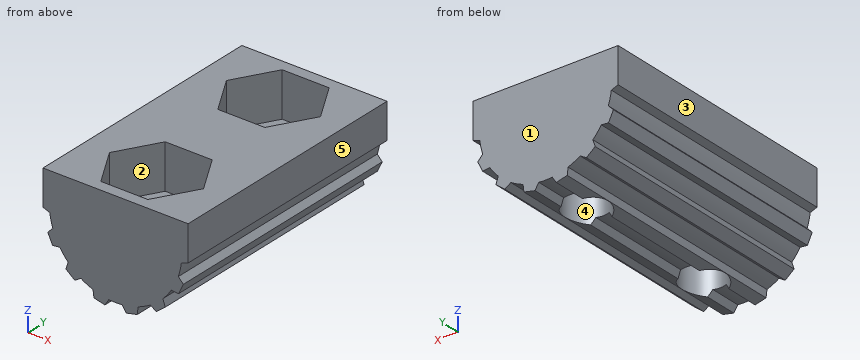
```python
from build123d import *

# Parameters (mm, degrees)
BOSS_EXTRUDE1_DEPTH             = 8.5
BOSS_EXTRUDE2_REACH             = 12.596
BOSS_EXTRUDE2_DIRECTION_2_REACH = 12.596
CIRPATTERN1_START               = -8.5
CIRPATTERN1_DEPTH               = 17
CUT_EXTRUDE1_DEPTH              = 19.347920123
CUT_EXTRUDE1_DEPTH_BACK         = 19.347920123
SKETCH10_W                      = 9.8
SKETCH10_H                      = 17
BOSS_EXTRUDE3_DEPTH             = 2
M2_5_CLEARANCE_HOLE1_D          = 2.9
CUT_EXTRUDE2_DEPTH              = 3


# Read off the part's stored shape, not the designer's step: CirPattern1
with BuildPart() as part:
    # Sketch1 → Boss-Extrude1 (new, symmetric)
    with BuildSketch(Plane(origin=(0, 0, 0), x_dir=(1, 0, 0), z_dir=(0, 1, 0))):
        with BuildLine():
            ThreePointArc((-4.44, 0.547426308), (-4.465207061, 0.274228857), (-4.473619962, 0))
            Line((-4.473619962, 0), (-4.44, 0))
            Line((-4.44, 0), (-4.44, 0.547426308))
        make_face()
        with BuildLine():
            Line((-4.44, 0.547426308), (-4.44, 0))
            Line((-4.44, 0), (4.473619962, 0))
            ThreePointArc((4.473619962, 0), (0.274228857, 4.465207061), (-4.44, 0.547426308))
        make_face()
    extrude(amount=BOSS_EXTRUDE1_DEPTH, both=True)

    # Boss-Extrude2: up to this face of the body (flat: up to its plane)
    boss_extrude2_end = Plane(part.part.faces().sort_by_distance((0, 8.5, -1.898663281))[0])
    # Sketch1<3> → Boss-Extrude2 (add, up to the picked face)
    with BuildSketch(Plane(origin=(0, 0, 0), x_dir=(1, 0, 0), z_dir=(0, 1, 0)), mode=Mode.PRIVATE) as boss_extrude2_sk1:
        Polygon((-4.44, 0.547426308), (-4.44, -0.547426308), (-4.9, -0.38), (-4.9, 0.38), align=None)
    boss_extrude2_tool1 = split(extrude(boss_extrude2_sk1.sketch, amount=BOSS_EXTRUDE2_REACH, mode=Mode.PRIVATE), bisect_by=boss_extrude2_end, keep=Keep.BOTH, mode=Mode.PRIVATE)
    # Sketch1<3> → Boss-Extrude2 (add, up to the picked face)
    with BuildSketch(Plane(origin=(0, 0, 0), x_dir=(1, 0, 0), z_dir=(0, 1, 0)), mode=Mode.PRIVATE) as boss_extrude2_sk2:
        with BuildLine():
            Line((-4.473619962, 0), (4.473619962, 0))
            ThreePointArc((4.473619962, 0), (0, 4.473619962), (-4.473619962, 0))
        make_face()
    boss_extrude2_tool2 = split(extrude(boss_extrude2_sk2.sketch, amount=BOSS_EXTRUDE2_REACH, mode=Mode.PRIVATE), bisect_by=boss_extrude2_end, keep=Keep.BOTH, mode=Mode.PRIVATE)
    add(boss_extrude2_tool1.solids().sort_by(Axis((-4.65616, 0, 0), (0, 1, 0)))[0])
    add(boss_extrude2_tool2.solids().sort_by(Axis((0, 0, -1.898663), (0, 1, 0)))[0])

    # Boss-Extrude2 direction 2: up to this face of the body (flat: up to its plane)
    boss_extrude2_direction_2_end = Plane(part.part.faces().sort_by_distance((0, -8.5, -1.898663281))[0])
    # Sketch1<3> → Boss-Extrude2 direction 2 (add, up to the picked face)
    with BuildSketch(Plane(origin=(0, 0, 0), x_dir=(1, 0, 0), z_dir=(0, 1, 0)), mode=Mode.PRIVATE) as boss_extrude2_direction_2_sk1:
        Polygon((-4.44, 0.547426308), (-4.44, -0.547426308), (-4.9, -0.38), (-4.9, 0.38), align=None)
    boss_extrude2_direction_2_tool1 = split(extrude(boss_extrude2_direction_2_sk1.sketch, amount=-BOSS_EXTRUDE2_DIRECTION_2_REACH, mode=Mode.PRIVATE), bisect_by=boss_extrude2_direction_2_end, keep=Keep.BOTH, mode=Mode.PRIVATE)
    # Sketch1<3> → Boss-Extrude2 direction 2 (add, up to the picked face)
    with BuildSketch(Plane(origin=(0, 0, 0), x_dir=(1, 0, 0), z_dir=(0, 1, 0)), mode=Mode.PRIVATE) as boss_extrude2_direction_2_sk2:
        with BuildLine():
            Line((-4.473619962, 0), (4.473619962, 0))
            ThreePointArc((4.473619962, 0), (0, 4.473619962), (-4.473619962, 0))
        make_face()
    boss_extrude2_direction_2_tool2 = split(extrude(boss_extrude2_direction_2_sk2.sketch, amount=-BOSS_EXTRUDE2_DIRECTION_2_REACH, mode=Mode.PRIVATE), bisect_by=boss_extrude2_direction_2_end, keep=Keep.BOTH, mode=Mode.PRIVATE)
    add(boss_extrude2_direction_2_tool1.solids().sort_by(Axis((-4.65616, 0, 0), (0, -1, 0)))[0])
    add(boss_extrude2_direction_2_tool2.solids().sort_by(Axis((0, 0, -1.898663), (0, -1, 0)))[0])

    # CirPattern1 outline → CirPattern1 (add)
    with BuildSketch(Plane(origin=(0, 0, 0), x_dir=(1, 0, 0), z_dir=(0, 1, 0)).offset(CIRPATTERN1_START)):
        with BuildLine():
            Line((4.9, 0.38), (4.44, 0.547426308))
            ThreePointArc((4.44, 0.547426308), (4.465207061, 0.274228857), (4.473619962, 0))
            ThreePointArc((4.473619962, 0), (4.465207061, -0.274228857), (4.44, -0.547426308))
            Line((4.44, -0.547426308), (4.9, -0.38))
            Line((4.9, -0.38), (4.9, 0.38))
        make_face()
        with BuildLine():
            Line((4.249871632, 2.468398491), (3.762782401, 2.419657862))
            ThreePointArc((3.762782401, 2.419657862), (4.030592313, 1.941030956), (4.237821147, 1.433229741))
            Line((4.237821147, 1.433229741), (4.579623274, 1.783662152))
            Line((4.579623274, 1.783662152), (4.249871632, 2.468398491))
        make_face()
        with BuildLine():
            Line((2.758004066, 4.067900389), (2.340299599, 3.812646502))
            ThreePointArc((2.340299599, 3.812646502), (2.789256424, 3.497616927), (3.196289842, 3.130017062))
            Line((3.196289842, 3.130017062), (3.352195992, 3.594048139))
            Line((3.352195992, 3.594048139), (2.758004066, 4.067900389))
        make_face()
        with BuildLine():
            Line((0.71987997, 4.861704725), (0.454291759, 4.450493744))
            ThreePointArc((0.454291759, 4.450493744), (0.995474092, 4.361456969), (1.521694134, 4.206866117))
            Line((1.521694134, 4.206866117), (1.460825183, 4.692588815))
            Line((1.460825183, 4.692588815), (0.71987997, 4.861704725))
        make_face()
        with BuildLine():
            Line((-1.460825183, 4.692588815), (-1.521694134, 4.206866117))
            ThreePointArc((-1.521694134, 4.206866117), (-0.995474092, 4.361456969), (-0.454291759, 4.450493744))
            Line((-0.454291759, 4.450493744), (-0.71987997, 4.861704725))
            Line((-0.71987997, 4.861704725), (-1.460825183, 4.692588815))
        make_face()
        with BuildLine():
            Line((-3.352195992, 3.594048139), (-3.196289842, 3.130017062))
            ThreePointArc((-3.196289842, 3.130017062), (-2.789256424, 3.497616927), (-2.340299599, 3.812646502))
            Line((-2.340299599, 3.812646502), (-2.758004066, 4.067900389))
            Line((-2.758004066, 4.067900389), (-3.352195992, 3.594048139))
        make_face()
        with BuildLine():
            Line((-3.7627824, 2.419657862), (-4.249871632, 2.468398491))
            Line((-4.249871632, 2.468398491), (-4.579623274, 1.783662152))
            Line((-4.579623274, 1.783662152), (-4.237821147, 1.433229741))
            ThreePointArc((-4.237821147, 1.433229741), (-4.030592312, 1.941030956), (-3.7627824, 2.419657862))
        make_face()
    extrude(amount=CIRPATTERN1_DEPTH)

    # Sketch4 → Cut-Extrude1 (cut, two sides: drawn at the far end of the back side and taken through both)
    with BuildSketch(Plane(origin=(0, 8.5, 0), x_dir=(1, 0, 0), z_dir=(0, 1, 0)).offset(-CUT_EXTRUDE1_DEPTH_BACK)):
        Polygon((-36.779321089, 0), (-4.9, 0), (4.9, 0), (36.779321089, 0), (36.779321089, -63.758642179), (-36.779321089, -63.758642179), align=None)
    extrude(amount=CUT_EXTRUDE1_DEPTH + CUT_EXTRUDE1_DEPTH_BACK, mode=Mode.SUBTRACT)

    # Sketch10 → Boss-Extrude3 (add)
    with BuildSketch(Plane.XY):
        Rectangle(SKETCH10_W, SKETCH10_H)
    extrude(amount=BOSS_EXTRUDE3_DEPTH)

    # M2.5 Clearance Hole1 (through all)
    with Locations(Plane(origin=(-2.188156234, 1.776538328, 2), x_dir=(1, 0, 0), z_dir=(0, 0, 1))):
        with Locations((2.188156234, 3.223461672), (2.188156234, -6.776538328)):
            Hole(M2_5_CLEARANCE_HOLE1_D / 2)

    # Sketch9 → Cut-Extrude2 (cut)
    with BuildSketch(Plane.XY.offset(2)):
        Polygon((-3.175426481, 5), (-1.58771324, 2.25), (1.58771324, 2.25), (3.175426481, 5), (1.58771324, 7.75), (-1.58771324, 7.75), align=None)
        Polygon((-3.175426481, -5), (-1.58771324, -7.75), (1.58771324, -7.75), (3.175426481, -5), (1.58771324, -2.25), (-1.58771324, -2.25), align=None)
    extrude(amount=-CUT_EXTRUDE2_DEPTH, mode=Mode.SUBTRACT)


solid = part.part
```
Can you work these out from the model? Positions are in its coordinate system, mm. Face numbers are marked on the shaded views. A direction names the side the tool comes from. Round coordinates to 2 decimals unless told otherwise and drop trailing zeros. Loops run counter-clockwise (first coordinate to the right, second up) from the corner with the lowest first, then second, coordinate; pieces in that order, holes last. Notation, with made-up numbers: M 31,-10 L 74,-10 A21 ccw 74,4 Z; hole C 25,-11.5 d10. An arc over 180 degrees is marked long. Write item = value, one per line. Start each with the question number.
(1) If we mould it in two halves opening along X, with no side actions, what happens to the marked faces 3, 4 and 5? For each: released by +X, released by -X, zero draft, split by the parting line, or undercut.
(2) Suppose I cut it at C-C on z = 0. Write out the boundary of the cut face in (x, y).
(3) Which directions (+Z, -Z, +X, -X, +Y, -Y) give clear straight access to the entire face, cutting with the end or side of a thin tool? Please do the marked faces 1 and 2.
(4) Suppose I cut it at D-D on x = 1. Write out the boundary of the cut face in (y, z), plus the area to 3 significant figures.
(5) I'm going to push flat-ended pins straight in: P1, Ø2, axis at y = 1, z = -3.5, coming from the -X side; P2, Ø2, axis at y = -1.5, z = -2.5, coming from the -X side; P3, Ø2.5, axis at x = 0, y = 5, coming from the +Z side. Where does each tip first touch, or does it pass through?
(6) I need wall thicknesses on line 1 along Y through (x, z) = (0, -2.9); line 2 along Y through (x, z) = (0.25, 1.5); line 3 along X through (y, z) = (1, -4). Which ranges of each line are inside material? Lowest first, please.
(7) Suppose I cut it at A-A on x = 0. Write out the boundary of the cut face in (y, z).
Answer block:
q1.face_3 = released by -X
q1.face_4 = undercut
q1.face_5 = released by +X
q2.outline = M -4.9,-8.5 L 4.9,-8.5 L 4.9,8.5 L -4.9,8.5 Z; hole M -3.18,-5 L -1.59,-7.75 L 1.59,-7.75 L 3.18,-5 L 1.59,-2.25 L -1.59,-2.25 Z; hole M -3.18,5 L -1.59,2.25 L 1.59,2.25 L 3.18,5 L 1.59,7.75 L -1.59,7.75 Z
q3.face_1 = +Z, -Z, +X, -X, +Y
q3.face_2 = +Z
q4.outline = M -8.5,-4.8 L -6.05,-4.8 L -6.05,-1 L -7.75,-1 L -7.75,2 L -8.5,2 Z; M -3.95,-4.8 L 3.95,-4.8 L 3.95,-1 L 2.25,-1 L 2.25,2 L -2.25,2 L -2.25,-1 L -3.95,-1 Z; M 6.05,-4.8 L 8.5,-4.8 L 8.5,2 L 7.75,2 L 7.75,-1 L 6.05,-1 Z
q4.area = 66.6 mm²
q5.P1 = -3.71
q5.P2 = -4.58
q5.P3 = through
q6.line_1 = -8.5 to -6.45, -3.55 to 3.55, 6.45 to 8.5
q6.line_2 = -8.5 to -7.75, -2.25 to 2.25, 7.75 to 8.5
q6.line_3 = -2.84 to -2.65, -2 to 2, 2.65 to 2.84
q7.outline = M -8.5,-4.47 L -6.45,-4.47 L -6.45,-1 L -7.75,-1 L -7.75,2 L -8.5,2 Z; M -3.55,-4.47 L 3.55,-4.47 L 3.55,-1 L 2.25,-1 L 2.25,2 L -2.25,2 L -2.25,-1 L -3.55,-1 Z; M 6.45,-4.47 L 8.5,-4.47 L 8.5,2 L 7.75,2 L 7.75,-1 L 6.45,-1 Z
